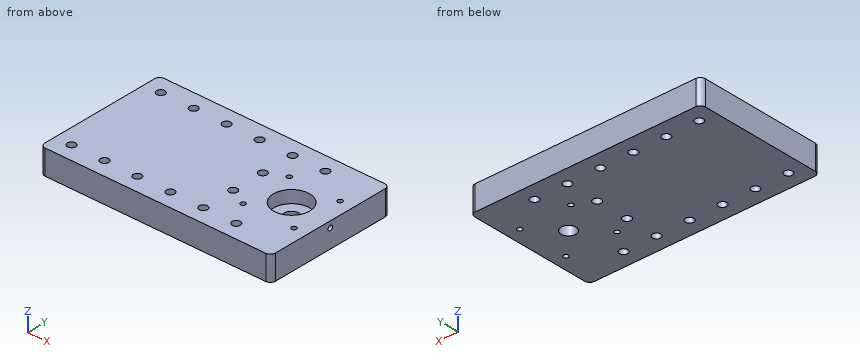
```python
from build123d import *

# Parameters (mm, degrees)
SKETCH1_W               = 60
SKETCH1_H               = 80
SKETCH1_R               = 1.5
SKETCH1_R_2             = 11
SKETCH1_R_3             = 2.5
SKETCH1_W_2             = 80
BOSS_EXTRUDE1_DEPTH     = 15
SKETCH1_3_R             = 11
SKETCH1_3_R_2           = 4.5
BOSS_EXTRUDE2_DEPTH     = 7.5
FILLET1_R               = 3
CUT_EXTRUDE1_REACH      = 163.941
CUT_EXTRUDE1_END_RADIUS = 11
SKETCH2_R               = 1.5


with BuildPart() as part:
    # Sketch1 → Boss-Extrude1 (new body)
    # profile 1 of 2: a face of its own
    with BuildSketch(Plane.XY):
        with Locations((30, 40)):
            Rectangle(SKETCH1_W, SKETCH1_H)
        with Locations((21, 24.5)):
            Circle(SKETCH1_R, mode=Mode.SUBTRACT)
        with Locations((52, 24.5)):
            Circle(SKETCH1_R, mode=Mode.SUBTRACT)
        with Locations((52, 55.5)):
            Circle(SKETCH1_R, mode=Mode.SUBTRACT)
        with Locations((21, 55.5)):
            Circle(SKETCH1_R, mode=Mode.SUBTRACT)
        with Locations((36.5, 40)):
            Circle(SKETCH1_R_2, mode=Mode.SUBTRACT)
        with Locations((30, 10)):
            Circle(SKETCH1_R_3, mode=Mode.SUBTRACT)
        with Locations((30, 70)):
            Circle(SKETCH1_R_3, mode=Mode.SUBTRACT)
        with Locations((10, 70)):
            Circle(SKETCH1_R_3, mode=Mode.SUBTRACT)
        with Locations((10, 50)):
            Circle(SKETCH1_R_3, mode=Mode.SUBTRACT)
        with Locations((10, 30)):
            Circle(SKETCH1_R_3, mode=Mode.SUBTRACT)
        with Locations((10, 10)):
            Circle(SKETCH1_R_3, mode=Mode.SUBTRACT)
    # profile 2 of 2: a face of its own
    with BuildSketch(Plane.XY):
        with Locations((-40, 40)):
            Rectangle(SKETCH1_W_2, SKETCH1_H)
        with Locations((-10, 10)):
            Circle(SKETCH1_R_3, mode=Mode.SUBTRACT)
        with Locations((-30, 10)):
            Circle(SKETCH1_R_3, mode=Mode.SUBTRACT)
        with Locations((-50, 10)):
            Circle(SKETCH1_R_3, mode=Mode.SUBTRACT)
        with Locations((-70, 10)):
            Circle(SKETCH1_R_3, mode=Mode.SUBTRACT)
        with Locations((-10, 70)):
            Circle(SKETCH1_R_3, mode=Mode.SUBTRACT)
        with Locations((-30, 70)):
            Circle(SKETCH1_R_3, mode=Mode.SUBTRACT)
        with Locations((-50, 70)):
            Circle(SKETCH1_R_3, mode=Mode.SUBTRACT)
        with Locations((-70, 70)):
            Circle(SKETCH1_R_3, mode=Mode.SUBTRACT)
    extrude(amount=BOSS_EXTRUDE1_DEPTH)

    # Sketch1<3> → Boss-Extrude2 (add)
    with BuildSketch(Plane.XY):
        with Locations((36.5, 40)):
            Circle(SKETCH1_3_R)
        with Locations((36.5, 40)):
            Circle(SKETCH1_3_R_2, mode=Mode.SUBTRACT)
    extrude(amount=BOSS_EXTRUDE2_DEPTH)

    # Fillet1
    fillet1_edges = [part.edges().sort_by_distance(p)[0] for p in [
        (-80, 0, 7.5),
        (-80, 80, 7.5),
        (60, 80, 7.5),
        (60, 0, 7.5),
    ]]
    fillet(fillet1_edges, radius=FILLET1_R)

    # Cut-Extrude1: up to this cylinder (the profile starts outside it)
    cut_extrude1_end = Plane(origin=(36.5, 40, 11.25), z_dir=(0, 0, -1)) * Cylinder(CUT_EXTRUDE1_END_RADIUS, 350.882, mode=Mode.PRIVATE)
    # Sketch2 → Cut-Extrude1 (cut, up to the surface)
    with BuildSketch(Plane(origin=(60, 0, 0), x_dir=(0, 0, -1), z_dir=(1, 0, 0)), mode=Mode.PRIVATE) as cut_extrude1_sk1:
        with Locations((-11.25, 40)):
            Circle(SKETCH2_R)
    cut_extrude1_tool1 = extrude(cut_extrude1_sk1.sketch, amount=-CUT_EXTRUDE1_REACH, mode=Mode.PRIVATE) - cut_extrude1_end
    add(cut_extrude1_tool1.solids().sort_by_distance((60, 40, 11.25))[0], mode=Mode.SUBTRACT)


solid = part.part
```
Input: part model. Units: mm. Frame: model coordinates. Coordinates: 2 decimals unless noted, no trailing zeros. Order: outer loops, then holes, each group sorted by start corner. A loop starts at its lowest first (then second) coordinate and runs counter-clockwise, first axis right, second up. Notation, with made-up numbers: (22.5, 22) - (70.5, 22) arc R18 ccw to (70.5, 29) - close; hole circle Ø9 at (32, 27.25). An arc over 180 degrees is marked (long way). Put each result on its own line as item: value.
1. Line query: line 1 along Y through (x, z) = (21, 4.75); line 2 along Y through (x, z) = (30, 4); line 3 along Y through (x, z) = (36.5, 2.25). Output: solid intervals per line, ascending.
Report:
line 1: y = 0 to 23, 26 to 54, 57 to 80
line 2: y = 0 to 7.5, 12.5 to 67.5, 72.5 to 80
line 3: y = 0 to 35.5, 44.5 to 80
2. Cut plane D-D on y = 24.5. Return the cut outline in (x, z).
Report:
outline: (-80, 0) - (19.5, 0) - (19.5, 15) - (-80, 15) - close; (22.5, 0) - (50.5, 0) - (50.5, 15) - (22.5, 15) - close; (53.5, 0) - (60, 0) - (60, 15) - (53.5, 15) - close
3. Cut plane A-A on x = 52. Return the cut outline in (y, z), then the cut area to 3 significant figures.
Report:
outline: (0, 0) - (23, 0) - (23, 15) - (0, 15) - close; (26, 0) - (54, 0) - (54, 15) - (26, 15) - close; (57, 0) - (80, 0) - (80, 15) - (57, 15) - close; hole circle Ø3 at (40, 11.25)
area: 1,100 mm2
4. Contact query for a flat-ended pin moving along its axis: pin 1 Ø11 at (x, y) = (37, 35) entering from +Z. Output: stop coordinate, or through.
Report:
pin 1: stops at z = 7.5
5. Cut plane B-B on z = 1.5. State how many separate pieces and enclosed holes the cut face has, then the cut area to 3 significant figures.
Report:
separate pieces: 1
enclosed holes: 19
area: 10,800 mm2
6. Cut plane C-C on y = 10. Return the cut outline in (x, z), then the cut area to 3 significant figures.
Report:
outline: (-80, 0) - (-72.5, 0) - (-72.5, 15) - (-80, 15) - close; (-67.5, 0) - (-52.5, 0) - (-52.5, 15) - (-67.5, 15) - close; (-47.5, 0) - (-32.5, 0) - (-32.5, 15) - (-47.5, 15) - close; (-27.5, 0) - (-12.5, 0) - (-12.5, 15) - (-27.5, 15) - close; (-7.5, 0) - (7.5, 0) - (7.5, 15) - (-7.5, 15) - close; (12.5, 0) - (27.5, 0) - (27.5, 15) - (12.5, 15) - close; (32.5, 0) - (60, 0) - (60, 15) - (32.5, 15) - close
area: 1,650 mm2
